The model under review builds one solid part; all positions refer to its coordinate system, in mm. A direction names the side the tool comes from. Give positions to 0.01 mm unless a question says otherwise; leave off trailing zeros. Order: outer loops, then holes, each group sorted by start corner. A loop starts at its lowest first (then second) coordinate and runs counter-clockwise, first axis right, second up. Notation, with made-up numbers: (25, 67.5) - (64, 67.5) arc R16 ccw to (64, 76.5) - close; hole circle Ø5 at (45.25, 59). An arc over 180 degrees is marked (long way). Use CSV: the item, a comma, the result in double quotes.
```python
from build123d import *

# Parameters (mm, degrees)
SKETCH_1_W      = 37
SKETCH_1_H      = 17
SKETCH_1_R      = 0.75
EXTRUDE_1_DEPTH = 1
SKETCH_1_3_W    = 10
SKETCH_1_3_H    = 10
EXTRUDE_2_DEPTH = 4
SKETCH_1_4_W    = 9.5
SKETCH_1_4_H    = 9.5
EXTRUDE_3_DEPTH = 5
SKETCH_1_5_W    = 4
SKETCH_1_5_H    = 2
EXTRUDE_4_DEPTH = 2


with BuildPart() as part:
    # Sketch 1 → Extrude 1 (new body)
    with BuildSketch(Plane(origin=(0, 0, 0), x_dir=(1, 0, 0), z_dir=(0, 1, 0))):
        Rectangle(SKETCH_1_W, SKETCH_1_H)
        with Locations(Location((-16.5, 4, 0), (0, 0, 270))):
            Circle(SKETCH_1_R, mode=Mode.SUBTRACT)
        with Locations(Location((-16.5, -4, 0), (0, 0, 270))):
            Circle(SKETCH_1_R, mode=Mode.SUBTRACT)
        with Locations(Location((16.5, -4, 0), (0, 0, 270))):
            Circle(SKETCH_1_R, mode=Mode.SUBTRACT)
        with Locations(Location((16.5, 4, 0), (0, 0, 270))):
            Circle(SKETCH_1_R, mode=Mode.SUBTRACT)
    extrude(amount=-EXTRUDE_1_DEPTH)

    # Sketch 1_3 → Extrude 2 (add)
    with BuildSketch(Plane(origin=(0, 0, 0), x_dir=(1, 0, 0), z_dir=(0, 1, 0))):
        with Locations((5.5, 2.5)):
            Rectangle(SKETCH_1_3_W, SKETCH_1_3_H)
    extrude(amount=EXTRUDE_2_DEPTH)

    # Sketch 1_4 → Extrude 3 (add)
    with BuildSketch(Plane(origin=(0, 0, 0), x_dir=(1, 0, 0), z_dir=(0, 1, 0))):
        with Locations((-7.25, -2.25)):
            Rectangle(SKETCH_1_4_W, SKETCH_1_4_H)
    extrude(amount=EXTRUDE_3_DEPTH)

    # Sketch 1_5 → Extrude 4 (add)
    with BuildSketch(Plane(origin=(0, 0, 0), x_dir=(1, 0, 0), z_dir=(0, 1, 0))):
        with Locations((-6.5, 6)):
            Rectangle(SKETCH_1_5_W, SKETCH_1_5_H)
    extrude(amount=EXTRUDE_4_DEPTH)


solid = part.part
```
Item 1: Clearance check with flat-ended pins moving along their axes: pin 1 (2 mm diameter, centred on x = -5, y = 2.5, fed in from +Z); pin 2 (2 mm diameter, centred on x = 16.5, z = -4, fed in from +Y); pin 3 (4 mm diameter, centred on x = 5, z = 2, fed in from +Y); pin 4 (0.9 mm diameter, centred on x = -16.5, z = -4, fed in from -Y). State where each tip first meets the part, or that it passes through.
Results list:
pin 1,"stops at z = 7"
pin 2,"stops at y = 0"
pin 3,"stops at y = 4"
pin 4,"passes through"
Item 2: Take a section at D-D, the plane x = 1. Give the boundary of the cut face in (y, z).
Results list:
outline,"(-1, -8.5) - (0, -8.5) - (0, -7.5) - (4, -7.5) - (4, 2.5) - (0, 2.5) - (0, 8.5) - (-1, 8.5) - close"
Item 3: Mouldability with a two-part tool opening along X and no side actions: class faces 6 (the face through (-4.5, 1, -6)), 7 (the face through (-7, 5, 2)), 8 (the face through (18.5, -0.5, 0.1)) as pulls with the +X half, pulls with the -X half, needs draft (parallel to the pull), parting line crosses it, or undercut.
Results list:
face 6,"undercut"
face 7,"needs draft"
face 8,"pulls with the +X half"
Item 4: Wall thickness on L1, parallel to X at y = -0.7, z = 4; L2, parallel to X at y = 3.25, z = 2; L3, parallel to Y at x = 12, z = 3: over which ranges is each line inside the solid? List them lowest first.
Results list:
L1,"x = -18.5 to -17.25, -15.75 to 15.75, 17.25 to 18.5"
L2,"x = -12 to -2.5, 0.5 to 10.5"
L3,"y = -1 to 0"
Item 5: Take a section at A-A, the plane y = 2.9. Give the boundary of the cut face in (x, z).
Results list:
outline,"(-12, -2.5) - (-2.5, -2.5) - (-2.5, 7) - (-12, 7) - close; (0.5, -7.5) - (10.5, -7.5) - (10.5, 2.5) - (0.5, 2.5) - close"
Item 6: Take a section at C-C, the plane x = 16.5. Give the boundary of the cut face in (y, z), and give its area (3 significant figures).
Results list:
outline,"(-1, -8.5) - (0, -8.5) - (0, -4.75) - (-1, -4.75) - close; (-1, -3.25) - (0, -3.25) - (0, 3.25) - (-1, 3.25) - close; (-1, 4.75) - (0, 4.75) - (0, 8.5) - (-1, 8.5) - close"
area,"14.0 mm2"
Item 7: Take a section at B-B, the plane z = -4. Give the boundary of the cut face in (x, y).
Results list:
outline,"(-18.5, -1) - (-17.25, -1) - (-17.25, 0) - (-18.5, 0) - close; (-15.75, -1) - (15.75, -1) - (15.75, 0) - (10.5, 0) - (10.5, 4) - (0.5, 4) - (0.5, 0) - (-15.75, 0) - close; (17.25, -1) - (18.5, -1) - (18.5, 0) - (17.25, 0) - close"
Item 8: Tool access review of faces 1 (the face through (-7, 2, 7)), 2 (the face through (-12, 2, 2)), 3 (the face through (5, 4, -3)), 4 (the face through (-7, 2, -2.5)), 5 (the face through (-8.5, 1, -6)): name each direction out of +Z, -Z, +X, -X, +Y, -Y from which nothing blocks a thin tool from reaching the whole face with its end or side.
Results list:
face 1,"+Z, +X, -X, +Y"
face 2,"+Z, -Z, -X, +Y"
face 3,"+Z, -Z, +X, +Y"
face 4,"-X, +Y"
face 5,"-Z, -X, +Y"
